from build123d import *

# Parameters (mm, degrees)
F1_DEPTH = 3


# Not quite as in the source:
# - a feature names something its author has since deleted; it is built from what else it names


with BuildPart() as f1:
    # F0 (on Front) → F1 (new body)
    with BuildSketch(Plane.XZ):
        with BuildLine():
            Line((-1.5, 100), (-1.5, 120))
            Line((-1.5, 120), (-6, 120))
            add(Edge.make_bspline(
                [(-6, 120), (-13.1006129086, 120), (-20, 115.0061184168), (-20, 110)],
                knots=[0, 0, 0, 0, 0.5, 0.5, 0.5, 0.5], degree=3))
            add(Edge.make_bspline(
                [(-20, 110), (-20, 104.9938815832), (-13.1006129086, 99.9755263329), (-6, 100)],
                knots=[0.5, 0.5, 0.5, 0.5, 1, 1, 1, 1], degree=3))
            Line((-6, 100), (-1.5, 100))
        make_face()
        Polygon((-12, 68), (-6, 68), (-6, 90), (-12, 90), (-12, 86), (-7.5, 86), (-7.5, 84), (-12, 84), (-12, 80), (-7.5, 80), (-7.5, 78), (-12, 78), (-12, 74), (-7.5, 74), (-7.5, 72), (-12, 72), align=None)
        Polygon((-12, 46), (-6, 46), (-6, 68), (-12, 68), (-12, 64), (-7.5, 64), (-7.5, 62), (-12, 62), (-12, 58), (-7.5, 58), (-7.5, 56), (-12, 56), (-12, 52), (-7.5, 52), (-7.5, 50), (-12, 50), align=None)
        with BuildLine():
            Line((-12, 64), (-12, 68))
            Line((-12, 68), (-12, 72))
            ThreePointArc((-12, 72), (-16, 68), (-12, 64))
        make_face()
        with BuildLine():
            Line((12, 68), (12, 64))
            ThreePointArc((12, 64), (16, 68), (12, 72))
            Line((12, 72), (12, 68))
        make_face()
        Polygon((6, 90), (6, 46), (12, 46), (12, 50), (7.5, 50), (7.5, 52), (12, 52), (12, 56), (7.5, 56), (7.5, 58), (12, 58), (12, 62), (7.5, 62), (7.5, 64), (12, 64), (12, 68), (12, 72), (7.5, 72), (7.5, 74), (12, 74), (12, 78), (7.5, 78), (7.5, 80), (12, 80), (12, 84), (7.5, 84), (7.5, 86), (12, 86), (12, 90), align=None)
        with BuildLine():
            Line((1.5, 0), (60, 0))
            Line((60, 0), (60, 5))
            ThreePointArc((60, 5), (58.5355339059, 8.5355339059), (55, 10))
            Line((55, 10), (32, 10))
            ThreePointArc((32, 10), (13.6152236891, 17.6152236891), (6, 36))
            Line((6, 36), (6, 46))
            Line((6, 46), (6, 90))
            Line((6, 90), (6, 100))
            add(Edge.make_bspline(
                [(6, 120), (13.1006129086, 120), (26.8993870914, 110.0122368336), (13.1006129086, 99.9755263329), (6, 100)],
                knots=[0, 0, 0, 0, 0.5, 1, 1, 1, 1], degree=3))
            Line((6, 120), (1.5, 120))
            Line((1.5, 120), (-1.5, 120))
            Line((-1.5, 120), (-1.5, 100))
            Line((-1.5, 100), (-6, 100))
            Line((-6, 100), (-6, 90))
            Line((-6, 90), (-6, 68))
            Line((-6, 68), (-6, 46))
            Line((-6, 46), (-6, 36))
            ThreePointArc((-6, 36), (-13.6152236891, 17.6152236891), (-32, 10))
            Line((-32, 10), (-55, 10))
            ThreePointArc((-55, 10), (-58.5355339059, 8.5355339059), (-60, 5))
            Line((-60, 5), (-60, 0))
            Line((-60, 0), (-1.5, 0))
            Line((-1.5, 0), (-1.5, 60))
            Line((-1.5, 60), (1.5, 60))
            Line((1.5, 60), (1.5, 0))
        make_face()
    extrude(amount=F1_DEPTH)


solid = f1.part
The model under review builds one solid part; all positions refer to its coordinate system, in mm. A direction names the side the tool comes from. Round coordinates to 2 decimals unless told otherwise and drop trailing zeros. Write each loop counter-clockwise with the first axis right and the second up, starting at its lowest first coordinate (ties: lowest second). Pieces come first, ordered by that corner, then holes. Notation, with made-up numbers: (8, -7) - (67, -7) arc R17 ccw to (67, 20) - close; hole circle Ø2 at (87, 83.25). An arc over 180 degrees is marked (long way). One line per item, written item: value. Start each with the question number.
1. Consider section B-B on x = -50.5. Write out the cut boundary in (y, z).
2. Clearance check with flat-ended pins moving along their axes: P1, Ø1.5, axis at x = 9.5, y = -1, coming from the -Z side; P2, Ø1, axis at y = -1.5, z = 85, coming from the -X side; P3, Ø0.9, axis at x = -9.5, y = -1, coming from the +Z side; P4, Ø1.5, axis at x = 9.5, y = -1.5, coming from the +Z side. State where each tip first meets the part, or that it passes through.
3. To check wall thickness, follow L1, parallel to X at y = -2.15, z = 47.5; L2, parallel to X at y = -1.65, z = 82.5; L3, parallel to Z at x = 36, y = -1.2. State the ranges of each line that lie inside material, in increasing order. Write a range as from..to.
4. Machinability: for faces 1 (the face through (59, -1, 8)), 2 (the face through (9, -1, 46)), 3 (the face through (-10, -1, 52)), which of the approach directions +Z, -Z, +X, -X, +Y, -Y give a long, thin tool a straight path to every point of the face, cutting with its end or side? Answer none if there is none.
5. The part is to be moulded in two halves that separate along Z. For faces 4 (the face through (-31, -1, 0)), 5 (the face through (1.5, -1, 30)), 6 (the face through (-12, -1, 88)), 7 (the face through (10, -1, 50)), say which applies: released by +Z, released by -Z, zero draft, split by the parting line, or undercut.
6. Consider section C-C on x = -14.5. State how many separate pieces and enclosed holes the cut face has, and give its area (3 significant figures).
7. Consider section D-D on z = 68. Write out the cut boundary in (x, y), and give its area (3 significant figures).
8. Consider section A-A on z = 27. Write out the cut boundary in (x, y).
Checks:
1. outline: (-3, 0) - (0, 0) - (0, 10) - (-3, 10) - close
2. P1: stops at z = 0
2. P2: stops at x = -7.5
2. P3: stops at z = 119.7
2. P4: stops at z = 119.76
3. L1: x = -12..-1.5, 1.5..12
3. L2: x = -12..12
3. L3: z = 0..10
4. face 1: +Z, +X, +Y, -Y
4. face 2: +X, +Y, -Y
4. face 3: -X, +Y, -Y
5. face 4: released by -Z
5. face 5: zero draft
5. face 6: undercut
5. face 7: undercut
6. separate pieces: 3
6. enclosed holes: 0
6. area: 115 mm^2
7. outline: (-16, -3) - (16, -3) - (16, 0) - (-16, 0) - close
7. area: 96.0 mm^2
8. outline: (-7.61, -3) - (-1.5, -3) - (-1.5, 0) - (-7.61, 0) - close; (1.5, -3) - (7.61, -3) - (7.61, 0) - (1.5, 0) - close
